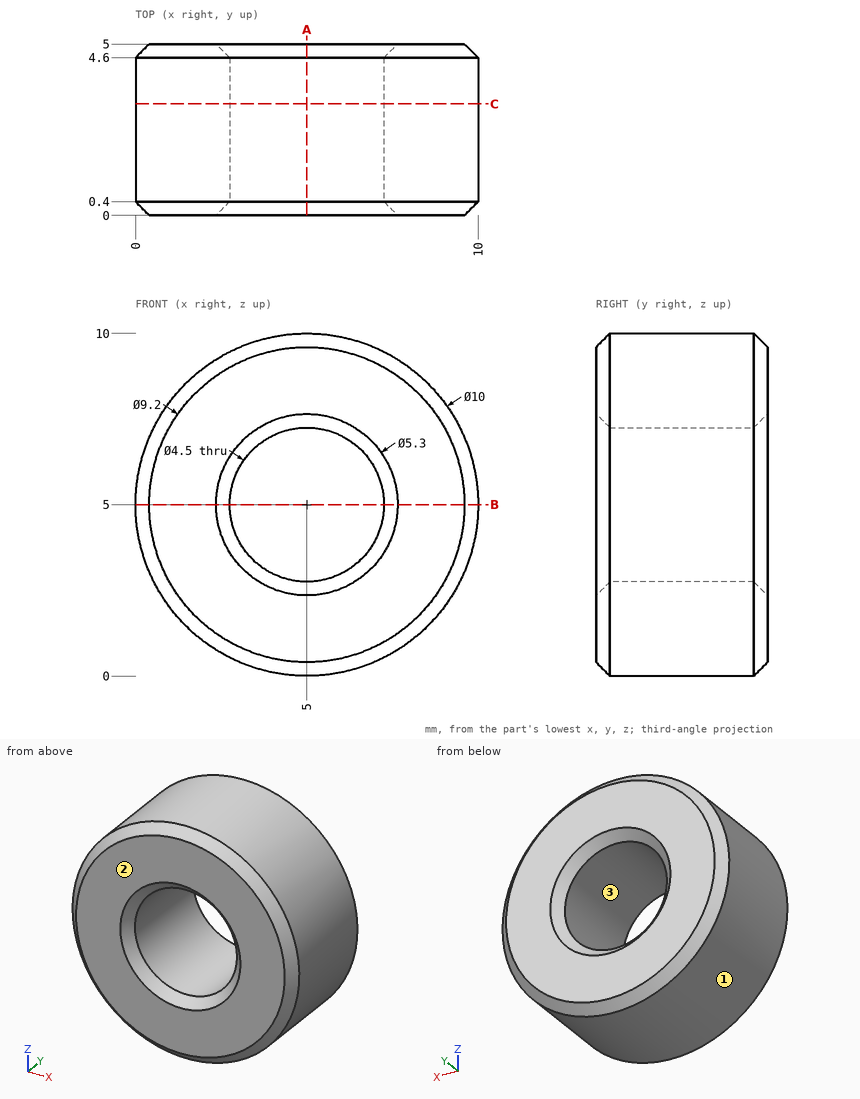
Source: three-view drawing plus pictorial views. Frame: mm from the lowest corner of the part. Give positions to 0.01 mm unless a question says otherwise; leave off trailing zeros. Order: outer loops, then holes, each group sorted by start corner. A loop starts at its lowest first (then second) coordinate and runs counter-clockwise, first axis right, second up. Notation, with made-up numbers: M 4,9.5 L 25,9.5 A19 ccw 25,25.5 Z; hole C -30,60.5 d8. An arc over 180 degrees is marked long. Return JSON: item names as keys, results as strings.
1) Mould query, pull axis Z, two halves, no side actions, for the marked faces 1, 2 and 3. Classes: released by +Z, released by -Z, zero draft, split by the parting line, or undercut.
Taken from the geometry:
{"face 1": "split by the parting line", "face 2": "zero draft", "face 3": "undercut"}
2) Contact query for a flat-ended pin moving along its axis: pin 1 (5 mm diameter, centred on x = 5, z = 5, fed in from +Y). Output: stop coordinate, or through.
Taken from the geometry:
{"pin 1": "stops at y = 4.85"}
3) Section query A-A on x = 5. Output: boundary loops of the cut face in (y, z).
Taken from the geometry:
{"outline": "M 0,0.4 L 0.4,0 L 4.6,0 L 5,0.4 L 5,2.35 L 4.6,2.75 L 0.4,2.75 L 0,2.35 Z; M 0,7.65 L 0.4,7.25 L 4.6,7.25 L 5,7.65 L 5,9.6 L 4.6,10 L 0.4,10 L 0,9.6 Z"}
4) Section query C-C on y = 3.25. Output: boundary loops of the cut face in (x, z).
Taken from the geometry:
{"outline": "C 5,5 d10; hole C 5,5 d4.5"}
5) Section query B-B on z = 5. Output: boundary loops of the cut face in (x, y).
Taken from the geometry:
{"outline": "M 0,0.4 L 0.4,0 L 2.35,0 L 2.75,0.4 L 2.75,4.6 L 2.35,5 L 0.4,5 L 0,4.6 Z; M 7.25,0.4 L 7.65,0 L 9.6,0 L 10,0.4 L 10,4.6 L 9.6,5 L 7.65,5 L 7.25,4.6 Z"}
6) Line query: L1, parallel to X at y = 3.5, z = 5; L2, parallel to Z at x = 4.75, y = 2.7; L3, parallel to Z at x = 3, y = 1.8. Output: solid intervals per line, ascending. Write a range as [from, to].
Taken from the geometry:
{"L1": "x = [0, 2.75], [7.25, 10]", "L2": "z = [0.01, 2.76], [7.24, 9.99]", "L3": "z = [0.42, 3.97], [6.03, 9.58]"}
